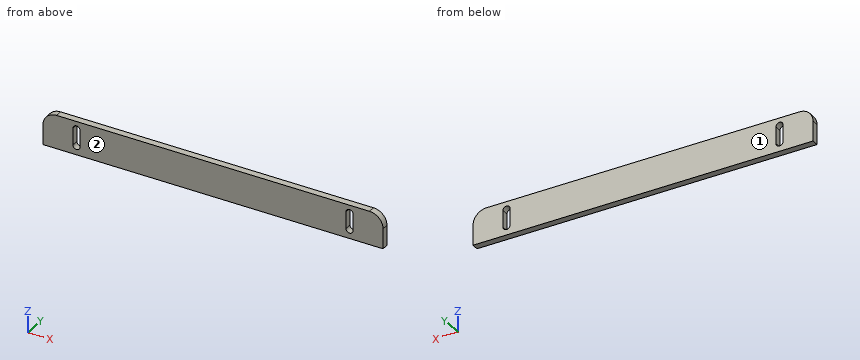
from build123d import *

# Parameters (mm, degrees)
SALIENTE_EXTRUIR1_DEPTH = 5


with BuildPart() as part:
    # Croquis1 → Saliente-Extruir1 (new body)
    with BuildSketch(Plane(origin=(0, 0, 0), x_dir=(1, 0, 0), z_dir=(0, 1, 0))):
        with BuildLine():
            Line((10, 0), (241, 0))
            ThreePointArc((241, 0), (248.071067812, 2.928932188), (251, 10))
            Line((251, 10), (251, 25))
            Line((251, 25), (0, 25))
            Line((0, 25), (0, 10))
            ThreePointArc((0, 10), (2.928932188, 2.928932188), (10, 0))
        make_face()
        with BuildLine():
            Line((27.395, 18.359540636), (27.395, 5.859540636))
            ThreePointArc((27.395, 5.859540636), (24.77, 3.234540636), (22.145, 5.859540636))
            Line((22.145, 5.859540636), (22.145, 18.359540636))
            ThreePointArc((22.145, 18.359540636), (24.77, 20.984540636), (27.395, 18.359540636))
        make_face(mode=Mode.SUBTRACT)
        with BuildLine():
            Line((223.605, 18.359540636), (223.605, 5.859540636))
            ThreePointArc((223.605, 5.859540636), (226.23, 3.234540636), (228.855, 5.859540636))
            Line((228.855, 5.859540636), (228.855, 18.359540636))
            ThreePointArc((228.855, 18.359540636), (226.23, 20.984540636), (223.605, 18.359540636))
        make_face(mode=Mode.SUBTRACT)
    extrude(amount=SALIENTE_EXTRUIR1_DEPTH)


solid = part.part
CAD build for the part. Positions are in the model's coordinates, mm. Face numbers are marked on the shaded views. Coordinates: 2 decimals unless noted, no trailing zeros. Write each loop counter-clockwise with the first axis right and the second up, starting at its lowest first coordinate (ties: lowest second). Pieces come first, ordered by that corner, then holes. Notation, with made-up numbers: M 25.5,-30.75 L 75.5,-30.75 A14 cw 75.5,-8.75 Z; hole C 53.5,79 d5. An arc over 180 degrees is marked long. Answer as a JSON object with one key per item and string values. Group by question number.
1) Wall check: line 1 (X direction, y = 1.5, z = -9.75) (3 decimals); line 2 (X direction, y = 1.8, z = -8.75) (3 decimals); line 3 (X direction, y = 4.15, z = -2.5). Give the ranges that are in metal, low to high. Write a range as from..to.
2) Mould opens along Y. For the marked faces 1 and 2 say: +Y half, -Y half, draft (parallel to the pull), parting line (faces both ways), or undercut.
3) Saw through at B-B (y = 4.25). Write the cut outline in (x, z) (3 decimals).
4) Saw through at A-A (x = 24.77). Write the cut outline in (y, z), plus the area to 4 significant figures.
Values follow:
{
 "1": {"line 1": "x = 0.003..22.145, 27.395..223.605, 228.855..250.997", "line 2": "x = 0.078..22.145, 27.395..223.605, 228.855..250.922", "line 3": "x = 3.39..247.61"},
 "2": {"face 1": "+Y half", "face 2": "-Y half"},
 "3": {"outline": "M 0,-25 L 251,-25 L 251,-10 A10 ccw 241,0 L 10,0 A10 ccw 0,-10 Z; hole M 22.145,-18.36 A2.625 ccw 27.395,-18.36 L 27.395,-5.86 A2.625 ccw 22.145,-5.86 Z; hole M 223.605,-18.36 A2.625 ccw 228.855,-18.36 L 228.855,-5.86 A2.625 ccw 223.605,-5.86 Z"},
 "4": {"outline": "M 0,-25 L 5,-25 L 5,-20.98 L 0,-20.98 Z; M 0,-3.23 L 5,-3.23 L 5,0 L 0,0 Z", "area": "36.25 mm2"}
}
